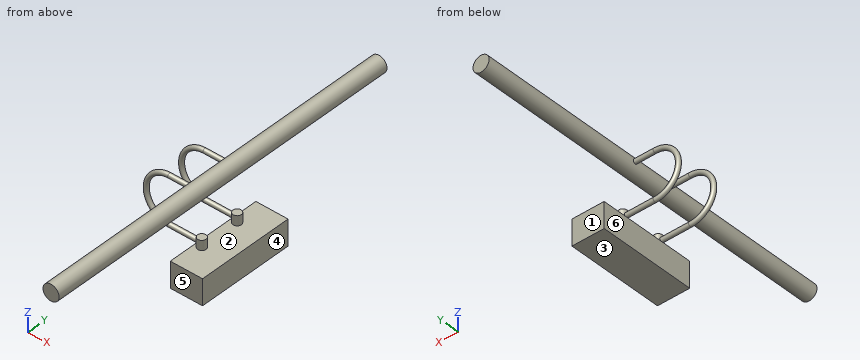
```python
from build123d import *

# Parameters (mm, degrees)
F0_W     = 50
F0_H     = 150
F1_DEPTH = 40
F2_R     = 6.5
F3_DEPTH = 15
F4_R     = 12.5
F5_DEPTH = 287.5
F9_R     = 3.5


with BuildPart() as f1:
    # F0 (on Top) → F1 (new body)
    with BuildSketch(Plane.XY):
        with Locations((-25, 0)):
            Rectangle(F0_W, F0_H)
    extrude(amount=F1_DEPTH)

    # F2 (on face) → F3 (join)
    with BuildSketch(Plane.XY.offset(40)):
        with Locations((-40, -31)):
            Circle(F2_R)
        with Locations((-40, 31)):
            Circle(F2_R)
    extrude(amount=F3_DEPTH)



with BuildPart() as f5:
    # F4 (on Front) → F5 (new body, symmetric)
    with BuildSketch(Plane.XZ):
        with Locations((-47, 120)):
            Circle(F4_R)
    extrude(amount=F5_DEPTH, both=True)


with BuildPart() as f1_1:
    add(f1.part)

    add(f5.part)  # F10 merges F5
    # F10: sweep along a path in F7
    with BuildLine(Plane.XZ.offset(31)) as f10_path:
        Line((-50, 120), (-90, 120))
        ThreePointArc((-90, 120), (-126.25, 83.75), (-90, 47.5))
        Line((-90, 47.5), (-40, 47.5))
    # F9 (on line) → F10 (sweep)
    with BuildSketch(Plane(origin=(-50, 0, 0), x_dir=(0, -1, 0), z_dir=(-1, 0, 0))):
        with Locations((31, 120)):
            Circle(F9_R)
    sweep(path=f10_path.line)

    # F11: F1 across plane


with BuildPart() as f1_2:
    add(f1_1.part)
    add(f1_1.part.mirror(Plane.XZ))


solid = f1_2.part
```
Input: part model. Units: mm. Frame: model coordinates. Face numbers are marked on the shaded views. A direction names the side the tool comes from. Coordinates: 2 decimals unless noted, no trailing zeros. Order: outer loops, then holes, each group sorted by start corner. A loop starts at its lowest first (then second) coordinate and runs counter-clockwise, first axis right, second up. Notation, with made-up numbers: (-3.75, 18) - (36.25, 18) arc R29 cw to (36.25, 53) - close; hole circle Ø5 at (50, -14.75). An arc over 180 degrees is marked (long way). Put each result on its own line as item: value.
1. Reachability of the marked faces 4, 5 and 6 from +Z, -Z, +X, -X, +Y, -Y: full face, straight path, thin tool, end or side. Return the list, or none.
Report:
face 4: +Z, -Z, +X, +Y, -Y
face 5: -Z, +X, -X, -Y
face 6: -Z, -X, +Y, -Y
2. Line query: line 1 along X through (y, z) = (-54.5, 15); line 2 along Z through (x, y) = (-27, 37); line 3 along Y through (x, z) = (-26, 13). Output: solid intervals per line, ascending.
Report:
line 1: x = -50 to 0
line 2: z = 0 to 40
line 3: y = -75 to 75
3. Cut plane C-C on x = -66.5. Return the cut outline in (y, z), then the cut area to 3 significant figures.
Report:
outline: circle Ø7 at (-31, 47.5); circle Ø7 at (-31, 120); circle Ø7 at (31, 47.5); circle Ø7 at (31, 120)
area: 154 mm2
4. Contact query for flat-ended pins moving along their axis: pin 1 Ø4 at (x, y) = (-38, -31.5) entering from +Z; pin 2 Ø5 at (x, y) = (-43, 225.5) entering from +Z; pin 3 Ø20 at (x, z) = (-35.5, 21.5) entering from -Y; pin 4 Ø12 at (x, z) = (-105, 65.5) entering from -Y. Output: stop coordinate, or through.
Report:
pin 1: stops at z = 130.36
pin 2: stops at z = 132.41
pin 3: stops at y = -75
pin 4: passes through
5. Cut plane A-A on y = -13. Return the cut outline in (x, z).
Report:
outline: circle Ø25 at (-47, 120); (-50, 0) - (0, 0) - (0, 40) - (-50, 40) - close
6. Cut plane D-D on y = 124. Return the cut outline in (x, z), then the cut area to 3 significant figures.
Report:
outline: circle Ø25 at (-47, 120)
area: 491 mm2
7. Draft query along Z for the marked faces 1, 2 and 3. Return one class per face: pulls with the +Z half, pulls with the -Z half, needs draft (parallel to the pull), parting line crosses it, or undercut.
Report:
face 1: needs draft
face 2: undercut
face 3: pulls with the -Z half
8. Cut plane B-B on x = -40. Return the cut outline in (y, z), then the cut area to 3 significant figures.
Report:
outline: (-287.5, 109.64) - (287.5, 109.64) - (287.5, 130.36) - (-287.5, 130.36) - close; (-75, 0) - (75, 0) - (75, 40) - (37.5, 40) - (37.5, 55) - (24.5, 55) - (24.5, 40) - (-24.5, 40) - (-24.5, 55) - (-37.5, 55) - (-37.5, 40) - (-75, 40) - close
area: 18,300 mm2
